For this review, take the finished solid that the model builds, in its own axes (mm). A direction names the side the tool comes from. Round coordinates to 2 decimals unless told otherwise and drop trailing zeros. Order: outer loops, then holes, each group sorted by start corner. A loop starts at its lowest first (then second) coordinate and runs counter-clockwise, first axis right, second up. Notation, with made-up numbers: M -21,52.5 L 15,52.5 A15 cw 15,79.5 Z; hole C 1.5,15 d9. An arc over 180 degrees is marked long. Answer as a JSON object with one key per item and string values.
from build123d import *

# Parameters (mm, degrees)
BOSS_EXTRUDE1_DEPTH = 6.35


with BuildPart() as part:
    # Sketch1 → Boss-Extrude1 (new body)
    with BuildSketch(Plane.XY):
        with BuildLine():
            Line((0, 0), (-4.3434, 0))
            ThreePointArc((-4.3434, 0), (-3.0734, 1.27), (-4.3434, 2.54))
            Line((-4.3434, 2.54), (-6.477, 2.54))
            ThreePointArc((-6.477, 2.54), (-7.274862364, 3.073114588), (-7.087657416, 4.014257416))
            Line((-7.087657416, 4.014257416), (-3.764962651, 7.336952181))
            ThreePointArc((-3.764962651, 7.336952181), (-2.730139224, 8.017998618), (-1.513461851, 8.2511937))
            Line((-1.513461851, 8.2511937), (0, 8.2511937))
            Line((0, 8.2511937), (0, 0))
        make_face()
    boss_extrude1 = extrude(amount=-BOSS_EXTRUDE1_DEPTH)

    # Mirror1: Boss-Extrude1 across plane
    add(boss_extrude1.mirror(Plane(origin=(0, 0, 0), x_dir=(0, 0, 1), z_dir=(1, 0, 0))))


solid = part.part
1) Add section B-B on y = 1.27. State the section outline as (x, z) points, and give its area (3 significant figures).
Geometry check:
{"outline": "M -3.07,-6.35 L 3.07,-6.35 L 3.07,0 L -3.07,0 Z", "area": "39.0 mm²"}
2) Mouldability with a two-part tool opening along Y and no side actions: class faces 1 (the cylindrical face through (7.27, 3.06, -3.13)), 2 (the cylindrical face through (-3.074, 1.242, -3.131)), 3 (the flat face through (0, 4, 0)) as +Y half, -Y half, draft (parallel to the pull), parting line (faces both ways), or undercut.
Geometry check:
{"face 1": "parting line", "face 2": "undercut", "face 3": "draft"}
3) Add section C-C on x = -5.5. State the section outline as (y, z) points, and give its area (3 significant figures).
Geometry check:
{"outline": "M 2.54,-6.35 L 5.6,-6.35 L 5.6,0 L 2.54,0 Z", "area": "19.4 mm²"}
4) Machinability: for faces 4 (the flat face through (-5, 2.54, -3)), 5 (the flat face through (5, 2.54, -3)), 6 (the flat face through (0, 0, -3)), which of the approach directions +Z, -Z, +X, -X, +Y, -Y give a long, thin tool a straight path to every point of the face, cutting with its end or side? Answer none if there is none.
Geometry check:
{"face 4": "+Z, -Z, -X, -Y", "face 5": "+Z, -Z, +X, -Y", "face 6": "+Z, -Z, +X, -X, -Y"}
5) For L1, parallel to X at y = 1.25, z = -1.25; L2, parallel to Y at x = 3.5, z = -0.5; L3, parallel to X at y = 5.75, z = -0.25, list the stretches that pass through material, from the lowest coordinate up.
Geometry check:
{"L1": "x = -3.07 to 3.07", "L2": "y = 0 to 0.32, 2.22 to 7.57", "L3": "x = -5.35 to 5.35"}
6) Insertion check: P1, Ø0.6, axis at x = 5, z = -3, coming from the -Y side; P2, Ø1, axis at y = 5, z = -2, coming from the +X side; P3, Ø1.5, axis at y = 5.5, z = -1.5, coming from the +X side. Each pin has a flat end and moves straight along its axis. Give the tip position at first contact, or say it passes through.
Geometry check:
{"P1": "stops at y = 2.54", "P2": "stops at x = 6.6", "P3": "stops at x = 6.35"}
7) Add section A-A on z = -4.5. State the section outline as (x, y) points (3 decimals).
Geometry check:
{"outline": "M -7.088,4.014 A0.864 ccw -6.477,2.54 L -4.343,2.54 A1.27 cw -4.343,0 L 4.343,0 A1.27 cw 4.343,2.54 L 6.477,2.54 A0.864 ccw 7.088,4.014 L 3.765,7.337 A3.175 ccw 1.513,8.251 L -1.513,8.251 A3.175 ccw -3.765,7.337 Z"}
